Verification items for this drawing (mm, ordinates from the low corner). A direction names the side the tool comes from. Round coordinates to 2 decimals unless told otherwise and drop trailing zeros. Loops run counter-clockwise (first coordinate to the right, second up) from the corner with the lowest first, then second, coordinate; pieces in that order, holes last. Notation, with made-up numbers: (22, 31) -> (46, 31) arc R37 cw to (46, 70) -> close; hole circle Ø4 at (5.5, 57.5). An arc over 180 degrees is marked (long way). Use a Markdown table: item, result. Add a question column.
Q1. Gauge pin test, flat ends, axial feed: P1, Ø1.5, axis at x = 63.5, z = 58, coming from the +Y side; P2, Ø8, axis at x = 126, y = 42, coming from the +Z side; P3, Ø2, axis at x = 16.5, y = 18.5, coming from the +Z side. Record the tip position at first contact, or that the pin passes through.
Q2. Sectioned sample at D-D, the plane y = 26.75. Give the number of separate pieces and of enclosed holes in the cut face.
Q3. Material ranges on L1, parallel to Z at x = 48, y = 13; L2, parallel to X at y = 74.5, z = 16 (1 decimal); L3, parallel to X at y = 59, z = 34.5 (1 decimal), recorded low to high.
Q4. Sectioned sample at B-B, the plane x = 134. Enter the section's corners in (y, z).
Q5. Sectioned sample at C-C, the plane z = 55. Enter the section's corners in (x, y) (1 decimal), then the cut area to 3 significant figures.
Q6. Set-up check for the marked faces 4 and 5: record each of +Z, -Z, +X, -X, +Y, -Y from which the full face is reachable in a straight line by a thin tool's end or side.
Q7. Release check for a two-part mould opening along Y. For the marked faces 1, 2 and 3 record: released by +Y, released by -Y, zero draft, split by the parting line, or undercut.
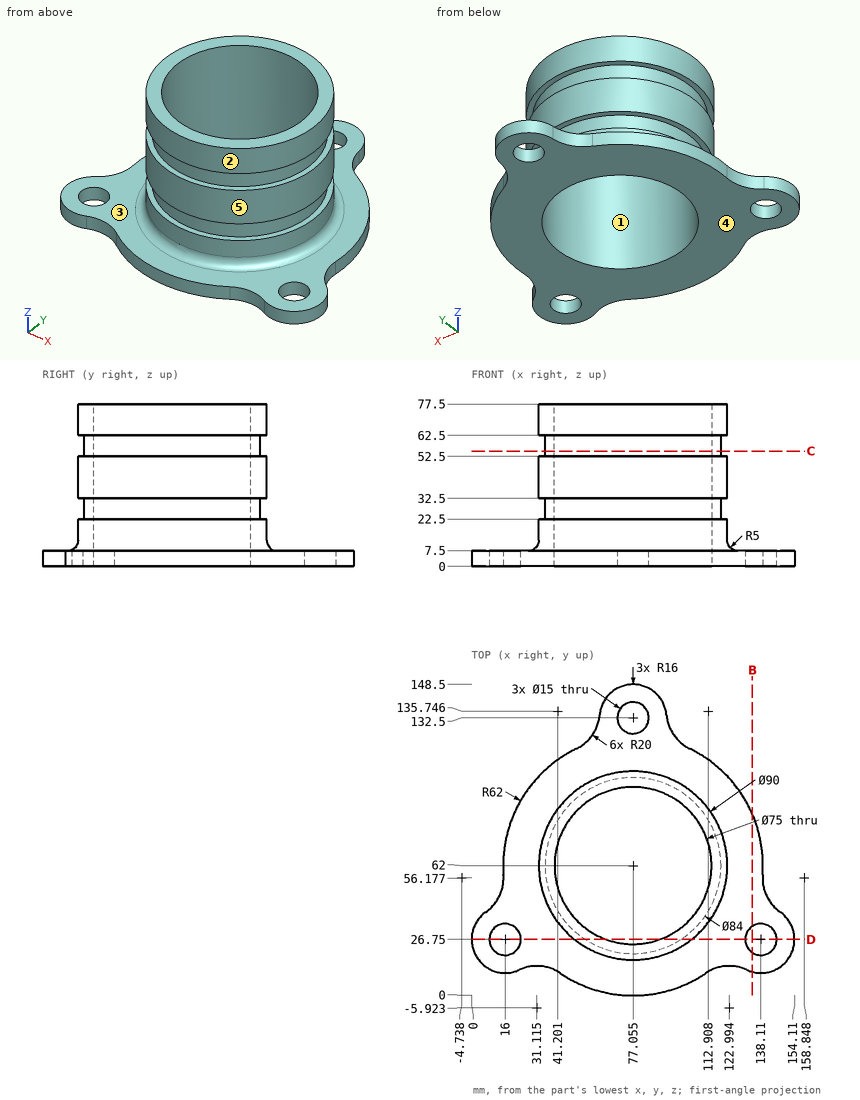
Values:
| question | item | result |
|---|---|---|
| 1 | P1 | y = 102 |
| 1 | P2 | z = 7.63 |
| 1 | P3 | z = 7.5 |
| 2 | separate pieces | 4 |
| 2 | enclosed holes | 0 |
| 3 | L1 | 0 to 7.5 |
| 3 | L2 | 33.8 to 41.7, 112.4 to 120.3 |
| 3 | L3 | 32.2 to 39.7, 114.4 to 122 |
| 4 | outline | (11.29, 0) -> (20.48, 0) -> (20.48, 7.5) -> (11.29, 7.5) -> close; (33.02, 0) -> (86.52, 0) -> (86.52, 7.5) -> (33.02, 7.5) -> close |
| 5 | outline | circle Ø84 at (77.1, 62); hole circle Ø75 at (77.1, 62) |
| 5 | area | 1,120 mm^2 |
| 6 | face 4 | -Z, +X, -X, +Y, -Y |
| 6 | face 5 | +Z |
| 7 | face 1 | undercut |
| 7 | face 2 | split by the parting line |
| 7 | face 3 | zero draft |
